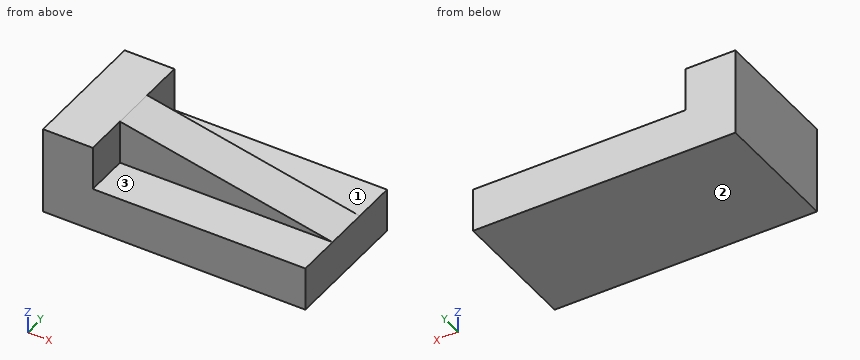
from build123d import *

# Parameters (mm, degrees)
F1_DEPTH = 76.2
F3_DEPTH = 76.2
F5_DEPTH = 25.4
F7_DEPTH = 25.4


with BuildPart() as f1:
    # F0 (on Front) → F1 (new body)
    with BuildSketch(Plane.XZ):
        Polygon((0, 50.8), (0, 0), (152.4, 0), (152.4, 25.4), (28.901575, 25.4), (28.901575, 50.8), align=None)
    extrude(amount=-F1_DEPTH)

    # F2 (on face) → F3 (join)
    with BuildSketch(Plane.XZ):
        Polygon((152.4, 25.4), (28.901575, 50.8), (28.901575, 25.4), align=None)
    extrude(amount=-F3_DEPTH)

    # F4 (on face) → F5 (cut)
    with BuildSketch(Plane.XZ):
        Polygon((152.4, 25.4), (28.901575, 50.8), (28.901575, 25.4), align=None)
    extrude(amount=-F5_DEPTH, mode=Mode.SUBTRACT)

    # F6 (on face) → F7 (cut)
    with BuildSketch(Plane(origin=(0, 76.2, 0), x_dir=(-1, 0, 0), z_dir=(0, 1, 0))):
        Polygon((-28.901575, 50.8), (-152.4, 25.4), (-28.901575, 25.4), align=None)
    extrude(amount=-F7_DEPTH, mode=Mode.SUBTRACT)


solid = f1.part
Verification items for the finished model (mm, model axes). Face numbers are marked on the shaded views. A direction names the side the tool comes from. Give positions to 0.01 mm unless a question says otherwise; leave off trailing zeros. Order: outer loops, then holes, each group sorted by start corner. A loop starts at its lowest first (then second) coordinate and runs counter-clockwise, first axis right, second up. Notation, with made-up numbers: (23.25, 22) -> (62.25, 22) arc R20 cw to (62.25, 45) -> close; hole circle Ø1 at (2, 61). An arc over 180 degrees is marked (long way). Answer as CSV lines item,"result".
Q1. Sectioned sample at D-D on y = 66. Record the cut outline in (x, z).
Solutions:
outline,"(0, 0) -> (152.4, 0) -> (152.4, 25.4) -> (28.9, 25.4) -> (28.9, 50.8) -> (0, 50.8) -> close"
Q2. Scan lines: probe 1 along Z at (x, y) = (42.5, 9); probe 2 along X at (y, z) = (9, 39); probe 3 along Y at (x, z) = (63.5, 28). Record each from-to range of solid material in increasing order.
Solutions:
probe 1,"z = 0 to 25.4"
probe 2,"x = 0 to 28.9"
probe 3,"y = 25.4 to 50.8"
Q3. Sectioned sample at B-B on x = 126. Record the cut outline in (y, z).
Solutions:
outline,"(0, 0) -> (76.2, 0) -> (76.2, 25.4) -> (50.8, 25.4) -> (50.8, 30.83) -> (25.4, 30.83) -> (25.4, 25.4) -> (0, 25.4) -> close"
Q4. Access from +Z, -Z, +X, -X, +Y, -Y to the whole of each face (thin tool, end or side, straight path). Record for the marked faces 1, 2 and 3.
Solutions:
face 1,"+Z, +X, +Y"
face 2,"-Z, +X, -X, +Y, -Y"
face 3,"+Z, +X, -Y"
Q5. Depth check by flat-ended pin: pin 1 (7.5 mm diameter, centred on x = 66.5, y = 67, fed in from +Z); pin 2 (10 mm diameter, centred on x = 137, y = 39, fed in from +Z); pin 3 (12.5 mm diameter, centred on y = 11.5, z = 39.5, fed in from +X). Enter the tip coordinate at first touch or a pass-through.
Solutions:
pin 1,"stops at z = 25.4"
pin 2,"stops at z = 29.6"
pin 3,"stops at x = 28.9"
Q6. Sectioned sample at A-A on y = 47. Record the cut outline in (x, z), plus the area to 3 significant figures.
Solutions:
outline,"(0, 0) -> (152.4, 0) -> (152.4, 25.4) -> (28.9, 50.8) -> (0, 50.8) -> close"
area,"6,170 mm²"
Q7. Sectioned sample at C-C on z = 45.5. Record the cut outline in (x, y), plus the area to 3 significant figures.
Solutions:
outline,"(0, 0) -> (28.9, 0) -> (28.9, 25.4) -> (54.67, 25.4) -> (54.67, 50.8) -> (28.9, 50.8) -> (28.9, 76.2) -> (0, 76.2) -> close"
area,"2,860 mm²"
